Work out the finished part from the listing and answer in its coordinate system (mm). Face numbers are marked on the shaded views. A direction names the side the tool comes from. Round coordinates to 2 decimals unless told otherwise and drop trailing zeros. Loops run counter-clockwise (first coordinate to the right, second up) from the corner with the lowest first, then second, coordinate; pieces in that order, holes last.
from build123d import *

# Parameters (mm, degrees)
BOSS_EXTRUDE1_DEPTH = 12.7
CIRPATTERN1_COUNT   = 3
SKETCH7_R           = 2.3
CUT_EXTRUDE2_DEPTH  = 6.35


with BuildPart() as part:
    # Sketch1 → Boss-Extrude1 (new body)
    with BuildSketch(Plane(origin=(0, 0, 0), x_dir=(1, 0, 0), z_dir=(0, 1, 0))):
        Polygon((11.547005384, -20), (23.094010768, 0), (11.547005384, 20), (-11.547005384, 20), (-23.094010768, 0), (-11.547005384, -20), align=None)
    extrude(amount=BOSS_EXTRUDE1_DEPTH)

    # Sketch5 → Cut-Revolve1 (revolve, cut)
    with BuildSketch(Plane(origin=(0, 12.7, 0), x_dir=(1, 0, 0), z_dir=(0, 1, 0))):
        Polygon((0, -20), (0, -4.792), (-3.81, -4.792), (-3.81, -10.888), (-11.176, -10.888), (-11.176, -18), (-6.5, -18), (-6.5, -20), align=None)
    cut_revolve1 = revolve(axis=Axis((0, 12.7, 20), (0, 0, -1)), mode=Mode.SUBTRACT)

    # CirPattern1: Cut-Revolve1 ×3 about axis
    cirpattern1_axis = Axis((0, 0, 0), (0, 1, 0))
    for i in range(1, CIRPATTERN1_COUNT):
        add(cut_revolve1.rotate(cirpattern1_axis, i * 360 / CIRPATTERN1_COUNT), mode=Mode.SUBTRACT)

    # Sketch7 → Cut-Extrude2 (cut)
    with BuildSketch(Plane(origin=(0, 12.7, 0), x_dir=(1, 0, 0), z_dir=(0, 1, 0))):
        with Locations((0, 14.700006)):
            Circle(SKETCH7_R)
        with Locations((12.730575168, -7.349997)):
            Circle(SKETCH7_R)
        with Locations((-12.730575168, -7.349997)):
            Circle(SKETCH7_R)
    extrude(amount=-CUT_EXTRUDE2_DEPTH, mode=Mode.SUBTRACT)


solid = part.part
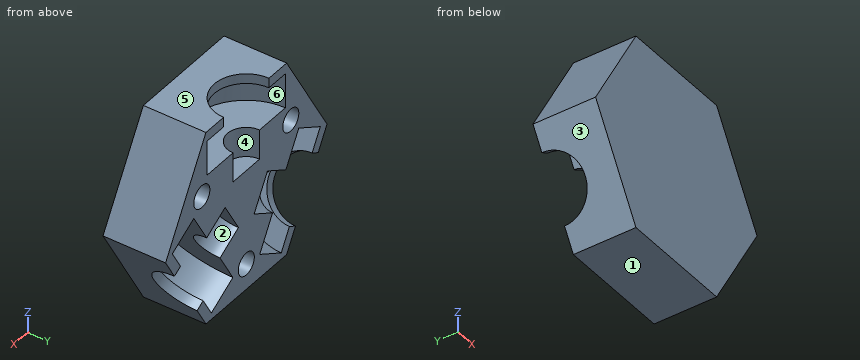
Item 1: Section A-A, the plane x = 0 is taken. Give the vertices of the cut face in (y, z), plus the area to 3 significant figures.
Item 2: Determine the mould class of the marked faces 1, 2 and 3 for opening direction X: pulls with the +X half, pulls with the -X half, needs draft (parallel to the pull), parting line crosses it, or undercut.
Item 3: For the marked faces 4, 5 and 6, determine the directions among +Z, -Z, +X, -X, +Y, -Y from which every point of the face is accessible in a straight line to the end or side of a thin tool.
Item 4: Section B-B, the plane y = 7.25 is taken. State how many separate pieces and enclosed holes the cut face has, plus the area to 3 significant figures.
Item 5: Each of these flat-tipped pins is pushed along its axis until it touches: P1, Ø4, axis at x = 0, z = -14.7, coming from the +Y side; P2, Ø4, axis at y = 7.5, z = -12.5, coming from the +X side; P3, Ø6, axis at x = -15.5, z = -5, coming from the +Y side. Where does it stop, or does it pass through?
Item 6: Straight lines are drawn through the part: line 1 (Z direction, x = -5, y = 4.5); line 2 (X direction, y = 7.5, z = -2.5); line 3 (X direction, y = 9.75, z = 2.5). For each, find the intervals that lie inside material, in ascending order.
Answer below:
1. outline: (0, -20) - (12.7, -20) - (12.7, -17) - (6.35, -17) - (6.35, -12.4) - (12.7, -12.4) - (12.7, 4.79) - (8.89, 4.79) - (8.89, 10.89) - (1.52, 10.89) - (1.52, 18) - (6.2, 18) - (6.2, 20) - (0, 20) - close
1. area: 363 mm2
2. face 1: needs draft
2. face 2: undercut
2. face 3: pulls with the -X half
3. face 4: +Z, +Y
3. face 5: +Z, +X, -X, +Y, -Y
3. face 6: +Y
4. separate pieces: 1
4. enclosed holes: 3
4. area: 877 mm2
5. P1: stops at y = 6.35
5. P2: stops at x = 16.79
5. P3: stops at y = 9.37
6. line 1: z = -20 to 10.89, 18 to 20
6. line 2: x = -21.65 to -19.34, -11.13 to 11.13, 19.34 to 21.65
6. line 3: x = -21.65 to -17.23, -14.02 to 14.02, 17.23 to 21.65
